Here's the drawing with two shaded views (mm, measured from the low corner). I have some questions. A direction names the side the tool comes from. Round coordinates to 2 decimals unless told otherwise and drop trailing zeros. Loops run counter-clockwise (first coordinate to the right, second up) from the corner with the lowest first, then second, coordinate; pieces in that order, holes last.
(1) Thinking about a two-plate mould opening in Z: for the marked faces 5, 6, 7 and 8, which applies, released by +Z, released by -Z, zero draft, split by the parting line, or undercut?
(2) I want a section at C-C on x = 29.5. Give the number of separate pieces and of enclosed holes in the cut face, plus the area to 3 significant figures.
(3) I want a section at A-A on y = 44. Write out the boundary of the cut face in (x, z).
(4) Which directions (+Z, -Z, +X, -X, +Y, -Y) give clear straight access to the entire face, cutting with the end or side of a thin tool? Please do the marked faces 1, 2, 3 and 4.
(5) I want a section at B-B on x = 76. Write out the boundary of the cut face in (y, z).
(6) Will these pins go through, and if not, where does the flat tip stop? pin 1 Ø3 at (x, y) = (52, 33.5) entering from +Z; pin 2 Ø1 at (y, z) = (48.5, 122.5) entering from +X; pin 3 Ø5 at (x, z) = (21.5, 142.5) entering from +Y.
(7) If I drill on line 1 along Z through (x, y) = (14, 38); line 2 along X through (y, z) = (45.5, 59); line 3 along Z through (x, y) = (56, 65.5), over which ranges is the centre line in solid material (lowest first)?
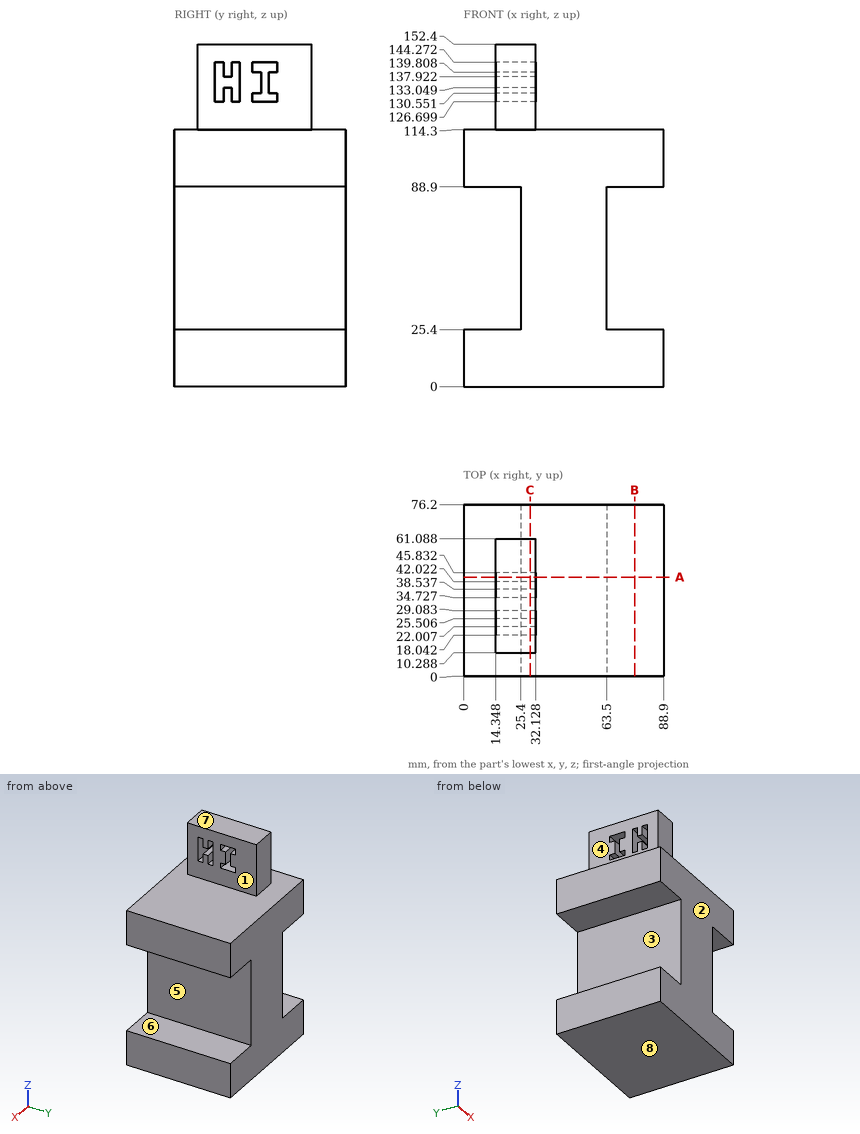
Filled sheet:
1. face 5: undercut
1. face 6: undercut
1. face 7: released by +Z
1. face 8: released by -Z
2. separate pieces: 1
2. enclosed holes: 2
2. area: 10,400 mm2
3. outline: (0, 0) - (88.9, 0) - (88.9, 25.4) - (63.5, 25.4) - (63.5, 88.9) - (88.9, 88.9) - (88.9, 114.3) - (32.13, 114.3) - (32.13, 126.7) - (14.35, 126.7) - (14.35, 114.3) - (0, 114.3) - (0, 88.9) - (25.4, 88.9) - (25.4, 25.4) - (0, 25.4) - close; (14.35, 130.55) - (32.13, 130.55) - (32.13, 139.81) - (14.35, 139.81) - close; (14.35, 144.27) - (32.13, 144.27) - (32.13, 152.4) - (14.35, 152.4) - close
4. face 1: +Z, +X, +Y, -Y
4. face 2: +Z, -Z, +X, -X, -Y
4. face 3: -X, +Y, -Y
4. face 4: +Z, -X, +Y, -Y
5. outline: (0, 0) - (76.2, 0) - (76.2, 25.4) - (0, 25.4) - close; (0, 88.9) - (76.2, 88.9) - (76.2, 114.3) - (0, 114.3) - close
6. pin 1: stops at z = 114.3
6. pin 2: stops at x = 32.13
6. pin 3: stops at y = 61.09
7. line 1: z = 0 to 25.4, 88.9 to 114.3
7. line 2: x = 25.4 to 63.5
7. line 3: z = 0 to 114.3
